Verification items for the finished model (mm, model axes). A direction names the side the tool comes from. Coordinates: 2 decimals unless noted, no trailing zeros. Order: outer loops, then holes, each group sorted by start corner. A loop starts at its lowest first (then second) coordinate and runs counter-clockwise, first axis right, second up.
Q1. Cross-section at B-B, the plane y = 14.5. Record the boundary of the cut face in (x, z).
Q2. Draft check along X on faces 1 (the flat face through (-2, 39.75, -8)), 2 (the cylindrical face through (-0.256, 37.74, -19.246)), 3 (the cylindrical face through (-4, 27, 26)), 4 (the flat face through (7.5, 27, 22)). Enter one of: pulls with the +X half, pulls with the -X half, needs draft (parallel to the pull), parting line crosses it, or undercut.
Q3. Cross-section at A-A, the plane z = 24.5. Record the boundary of the cut face in (x, y).
Q4. Thickness scan on line 1 (X direction, y = 27.1, z = -24.5); line 2 (X direction, y = 27, z = -24); line 3 (Z direction, x = 8, y = 22). Record the ranges inside material, lowest first.
Q5. Depth check by flat-ended pin: P1, Ø1.3, axis at y = 42, z = -10, coming from the -X side; P2, Ø5.5, axis at x = -4.5, z = 2, coming from the +Y side; P3, Ø1.6, axis at x = -3, y = 38, coming from the +Z side; P4, Ø2.5, axis at x = -4, z = -24.5, coming from the -Y side (1 decimal). Enter the tip coordinate at first touch or a pass-through.
Q6. Cross-section at C-C, the plane z = 16.5. Record the boundary of the cut face in (x, y), and give its area (4 significant figures).
Q7. Set-up check for faces 5 (the flat face through (0, 26, 23)), 6 (the cylindrical face through (1.802, 38.87, -4.277)), 7 (the flat face through (2, 41.2, -8.5)), 8 (the flat face through (-8.5, 38, 4)): record each of +Z, -Z, +X, -X, +Y, -Y from which the full face is reachable in a straight line by a thin tool's end or side.
Q8. Cross-section at D-D, the plane z = -20.5. Record the boundary of the cut face in (x, y).
from build123d import *

# Parameters (mm, degrees)
BOSS_EXTRUDE1_DEPTH = 37
BOSS_EXTRUDE2_DEPTH = 1.5
SKETCH4_R           = 6
BOSS_EXTRUDE3_DEPTH = 0.75
SKETCH5_R           = 4.5
BOSS_EXTRUDE4_DEPTH = 0.5
BOSS_EXTRUDE5_DEPTH = 3
SKETCH8_R           = 1.5
BOSS_EXTRUDE6_DEPTH = 2


with BuildPart() as part:
    # Sketch1 → Boss-Extrude1 (new body)
    with BuildSketch(Plane(origin=(0, 0, 0), x_dir=(1, 0, 0), z_dir=(0, 1, 0))):
        with BuildLine():
            Line((-8.25, 19.5), (8.25, 19.5))
            ThreePointArc((8.25, 19.5), (8.957106781, 19.207106781), (9.25, 18.5))
            Line((9.25, 18.5), (9.25, -18.5))
            ThreePointArc((9.25, -18.5), (8.957106781, -19.207106781), (8.25, -19.5))
            Line((8.25, -19.5), (-8.25, -19.5))
            ThreePointArc((-8.25, -19.5), (-8.957106781, -19.207106781), (-9.25, -18.5))
            Line((-9.25, -18.5), (-9.25, 18.5))
            ThreePointArc((-9.25, 18.5), (-8.957106781, 19.207106781), (-8.25, 19.5))
        make_face()
    extrude(amount=BOSS_EXTRUDE1_DEPTH)

    # Sketch3 → Boss-Extrude2 (add)
    with BuildSketch(Plane(origin=(0, 37, 0), x_dir=(1, 0, 0), z_dir=(0, 1, 0))):
        with BuildLine():
            Line((8.5, -13.5), (-8.5, -13.5))
            Line((-8.5, -13.5), (-8.5, 6.35137012))
            ThreePointArc((-8.5, 6.35137012), (0, 19.25), (8.5, 6.35137012))
            Line((8.5, 6.35137012), (8.5, -13.5))
        make_face()
    extrude(amount=BOSS_EXTRUDE2_DEPTH)

    # Sketch4 → Boss-Extrude3 (add)
    with BuildSketch(Plane(origin=(0, 38.5, 0), x_dir=(1, 0, 0), z_dir=(0, 1, 0))):
        with Locations(Location((0, 10, 0), (0, 0, 270))):
            Circle(SKETCH4_R)
    extrude(amount=BOSS_EXTRUDE3_DEPTH)

    # Sketch5 → Boss-Extrude4 (add)
    with BuildSketch(Plane(origin=(0, 39.25, 0), x_dir=(1, 0, 0), z_dir=(0, 1, 0))):
        with Locations(Location((0, 10, 0), (0, 0, 270))):
            Circle(SKETCH5_R)
    extrude(amount=BOSS_EXTRUDE4_DEPTH)

    # Sketch6 → Boss-Extrude5 (add)
    with BuildSketch(Plane(origin=(0, 39.75, 0), x_dir=(1, 0, 0), z_dir=(0, 1, 0))):
        Polygon((-2.5, 9.187700759), (-1.545084972, 7.873372979), (0, 7.371344439), (1.545084972, 7.873372979), (2.5, 9.187700759), (2.5, 10.812299241), (1.545084972, 12.126627021), (0, 12.628655561), (-1.545084972, 12.126627021), (-2.5, 10.812299241), align=None)
    extrude(amount=BOSS_EXTRUDE5_DEPTH)

    # Sketch8 → Boss-Extrude6 (add)
    # profile 1 of 2: a face of its own
    with BuildSketch(Plane(origin=(0, 26, 0), x_dir=(-1, 0, 0), z_dir=(0, -1, 0))):
        with BuildLine():
            ThreePointArc((-7.5, 25.5), (-7.207106781, 26.207106781), (-6.5, 26.5))
            Line((-6.5, 26.5), (6.5, 26.5))
            ThreePointArc((6.5, 26.5), (7.207106781, 26.207106781), (7.5, 25.5))
            Line((7.5, 25.5), (7.5, 19.5))
            Line((7.5, 19.5), (-7.5, 19.5))
            Line((-7.5, 19.5), (-7.5, 25.5))
        make_face()
        with Locations(Location((4, 24.5, 0), (0, 0, 90))):
            Circle(SKETCH8_R, mode=Mode.SUBTRACT)
        with Locations(Location((-4, 24.5, 0), (0, 0, 90))):
            Circle(SKETCH8_R, mode=Mode.SUBTRACT)
    # profile 2 of 2: a face of its own
    with BuildSketch(Plane(origin=(0, 26, 0), x_dir=(-1, 0, 0), z_dir=(0, -1, 0))):
        with BuildLine():
            Line((-7.5, -19.5), (-7.5, -25.5))
            ThreePointArc((-7.5, -25.5), (-7.207106781, -26.207106781), (-6.5, -26.5))
            Line((-6.5, -26.5), (6.5, -26.5))
            ThreePointArc((6.5, -26.5), (7.207106781, -26.207106781), (7.5, -25.5))
            Line((7.5, -25.5), (7.5, -19.5))
            Line((7.5, -19.5), (-7.5, -19.5))
        make_face()
        with Locations(Location((-4, -24.5, 0), (0, 0, 90))):
            Circle(SKETCH8_R, mode=Mode.SUBTRACT)
        with Locations(Location((4, -24.5, 0), (0, 0, 90))):
            Circle(SKETCH8_R, mode=Mode.SUBTRACT)
    extrude(amount=-BOSS_EXTRUDE6_DEPTH)


solid = part.part
Check values:
1. outline: (-9.25, -18.5) arc R1 ccw to (-8.25, -19.5) - (8.25, -19.5) arc R1 ccw to (9.25, -18.5) - (9.25, 18.5) arc R1 ccw to (8.25, 19.5) - (-8.25, 19.5) arc R1 ccw to (-9.25, 18.5) - close
2. face 1: needs draft
2. face 2: parting line crosses it
2. face 3: undercut
2. face 4: pulls with the +X half
3. outline: (-7.5, 26) - (-5.5, 26) - (-5.5, 28) - (-7.5, 28) - close; (-2.5, 26) - (2.5, 26) - (2.5, 28) - (-2.5, 28) - close; (5.5, 26) - (7.5, 26) - (7.5, 28) - (5.5, 28) - close
4. line 1: x = -7.5 to -5.5, -2.5 to 2.5, 5.5 to 7.5
4. line 2: x = -7.5 to -5.41, -2.59 to 2.59, 5.41 to 7.5
4. line 3: z = -19.5 to 19.5
5. P1: stops at x = -2.5
5. P2: stops at y = 38.5
5. P3: stops at z = 13.5
5. P4: passes through
6. outline: (-9.25, 0) - (9.25, 0) - (9.25, 37) - (-9.25, 37) - close
6. area: 684.5 mm2
7. face 5: +Z, +X, -X, -Y
7. face 6: +Y
7. face 7: +Z, +X, +Y
7. face 8: +Z, -X, +Y
8. outline: (-7.5, 26) - (7.5, 26) - (7.5, 28) - (-7.5, 28) - close
